from build123d import *

# Parameters (mm, degrees)
BOSS_EXTRUDE1_DEPTH = 2
SKETCH1_3_W         = 70
SKETCH1_3_H         = 43
BOSS_EXTRUDE2_DEPTH = 4
SKETCH1_5_W         = 40
SKETCH1_5_H         = 24
CUT_EXTRUDE4_DEPTH  = 2
CUT_EXTRUDE5_REACH  = 81.505
SKETCH2_W           = 39
SKETCH2_H           = 1.5
BOSS_EXTRUDE3_START = -0.5
BOSS_EXTRUDE3_DEPTH = 0.6
FILLET1_R           = 1


with BuildPart() as part:
    # Sketch1 → Boss-Extrude1 (new body)
    with BuildSketch(Plane(origin=(0, 0, 0), x_dir=(1, 0, 0), z_dir=(0, 1, 0))):
        Polygon((0, 0), (64, 0), (66, 0), (66, -1), (66, -38), (66, -39), (64, -39), (0, -39), align=None)
    extrude(amount=BOSS_EXTRUDE1_DEPTH)

    # Sketch1<3> → Boss-Extrude2 (add)
    with BuildSketch(Plane(origin=(0, 0, 0), x_dir=(1, 0, 0), z_dir=(0, 1, 0))):
        with Locations((33, -19.5)):
            Rectangle(SKETCH1_3_W, SKETCH1_3_H)
        Polygon((0, 0), (64, 0), (66, 0), (66, -1), (66, -38), (66, -39), (64, -39), (0, -39), align=None, mode=Mode.SUBTRACT)
    extrude(amount=BOSS_EXTRUDE2_DEPTH)

    # Sketch1<5> → Cut-Extrude4 (cut)
    with BuildSketch(Plane(origin=(0, 0, 0), x_dir=(1, 0, 0), z_dir=(0, 1, 0))):
        with Locations((20, -27)):
            Rectangle(SKETCH1_5_W, SKETCH1_5_H)
        with BuildLine():
            ThreePointArc((40, -15), (52, -27), (40, -39))
            Line((40, -39), (40, -15))
        make_face()
    extrude(amount=CUT_EXTRUDE4_DEPTH, mode=Mode.SUBTRACT)

    # Sketch2 → Cut-Extrude5 (cut, up to next)
    with BuildSketch(Plane(origin=(0, 0, 0), x_dir=(0, 0, -1), z_dir=(1, 0, 0)), mode=Mode.PRIVATE) as cut_extrude5_sk1:
        with Locations((-19.5, 3.25)):
            Rectangle(SKETCH2_W, SKETCH2_H)
    cut_extrude5_tool1 = extrude(cut_extrude5_sk1.sketch, amount=-CUT_EXTRUDE5_REACH, mode=Mode.PRIVATE) & part.part
    add(cut_extrude5_tool1.solids().sort_by_distance((0, 3.25, 19.5))[0], mode=Mode.SUBTRACT)

    # Sketch3 → Boss-Extrude3 (add)
    with BuildSketch(Plane(origin=(0, 4, 0), x_dir=(1, 0, 0), z_dir=(0, 1, 0)).offset(BOSS_EXTRUDE3_START)):
        Polygon((-2, -41), (68, -41), (68, 2), (-2, 2), (-2, -1), (65, -1), (65, -38), (-2, -38), align=None)
    extrude(amount=BOSS_EXTRUDE3_DEPTH)

    # Fillet1
    fillet1_edges = [part.edges().sort_by_distance(p)[0] for p in [
        (68, 2.05, -2),
        (-2, 0, 19.5),
        (-2, 2.05, -2),
        (33, 0, 41),
        (-2, 2.05, 41),
        (68, 2.05, 41),
        (33, 0, -2),
        (68, 0, 19.5),
        (33, 4.1, 41),
        (68, 4.1, 19.5),
        (33, 4.1, -2),
    ]]
    fillet(fillet1_edges, radius=FILLET1_R)


solid = part.part
Work out the finished part from the listing and answer in its coordinate system (mm). A direction names the side the tool comes from. Round coordinates to 2 decimals unless told otherwise and drop trailing zeros. Write each loop counter-clockwise with the first axis right and the second up, starting at its lowest first coordinate (ties: lowest second). Pieces come first, ordered by that corner, then holes. Notation, with made-up numbers: (77, 25.25) - (96, 25.25) arc R17 cw to (96, 55.25) - close; hole circle Ø7 at (-13.75, 71.5). An arc over 180 degrees is marked (long way). Answer in a Markdown table with one row per item. Add a question column.
1. Given pin 1 (0.5 mm diameter, centred on x = 41, y = 4, fed in from +Z); pin 2 (1.6 mm diameter, centred on x = -1, z = 23.5, fed in from +Y); pin 3 (11.5 mm diameter, centred on x = 16.5, z = 19.5, fed in from +Y), each flat-ended and moving along its own axis, determine where each tip first touches the part or whether it passes through.
2. The mould has two halves that part along X. Classify faces 4 (the flat face through (-2, 2, 20)), 5 (the flat face through (43, 4.1, 39)), 6 (the flat face through (32, 3, 0)): +X half, -X half, draft (parallel to the pull), parting line (faces both ways), or undercut.
3. A cutting plane is placed at A-A, the plane z = 27. Determine the outline of the cut face in (x, y), and give its area (3 significant figures).
4. A cutting plane is placed at C-C, the plane z = 12. Determine the outline of the cut face in (x, y).
5. For faces 1 (the flat face through (31.8, 3.5, 0.6)), 2 (the flat face through (66, 3, 19)), 3 (the flat face through (20, 1, 15)), determine the directions among +Z, -Z, +X, -X, +Y, -Y from which every point of the face is accessible in a straight line to the end or side of a thin tool.
6. Find the intervals of material crossed by line 1 along Z through (x, y) = (2, 0.85); line 2 along Z through (x, y) = (17.5, 3.05); line 3 along Y through (x, z) = (51.5, 8.5), in increasing order. Write a range as from..to.
7. A cutting plane is placed at D-D, the plane x = 44.5. Determine the outline of the cut face in (y, z).
8. A cutting plane is placed at B-B, the plane x = 11. Determine the outline of the cut face in (y, z), and give its area (3 significant figures).
Worked out:
| question | item | result |
|---|---|---|
| 1 | pin 1 | z = 40.76 |
| 1 | pin 2 | y = 2.5 |
| 1 | pin 3 | y = 2 |
| 2 | face 4 | -X half |
| 2 | face 5 | draft |
| 2 | face 6 | undercut |
| 3 | outline | (-2, 1) arc R1 ccw to (-1, 0) - (0, 0) - (0, 2.5) - (-2, 2.5) - close; (52, 0) - (67, 0) arc R1 ccw to (68, 1) - (68, 3.1) arc R1 ccw to (67, 4.1) - (65, 4.1) - (65, 3.5) - (66, 3.5) - (66, 2) - (52, 2) - close |
| 3 | area | 41.2 mm^2 |
| 4 | outline | (-2, 1) arc R1 ccw to (-1, 0) - (67, 0) arc R1 ccw to (68, 1) - (68, 3.1) arc R1 ccw to (67, 4.1) - (65, 4.1) - (65, 3.5) - (66, 3.5) - (66, 2) - (0, 2) - (0, 2.5) - (-2, 2.5) - close |
| 5 | face 1 | -X |
| 5 | face 2 | none |
| 5 | face 3 | +Y, -Y |
| 6 | line 1 | -1.99..15, 39..40.99 |
| 6 | line 2 | -2..0, 39..41 |
| 6 | line 3 | 0..2 |
| 7 | outline | (0, -1) arc R1 ccw to (1, -2) - (3.1, -2) arc R1 ccw to (4.1, -1) - (4.1, 1) - (3.5, 1) - (3.5, 0) - (2, 0) - (2, 15.88) - (0, 15.88) - close; (0, 38.12) - (2, 38.12) - (2, 39) - (3.5, 39) - (3.5, 38) - (4.1, 38) - (4.1, 40) arc R1 ccw to (3.1, 41) - (1, 41) arc R1 ccw to (0, 40) - close |
| 8 | outline | (0, -1) arc R1 ccw to (1, -2) - (3.1, -2) arc R1 ccw to (4.1, -1) - (4.1, 1) - (3.5, 1) - (3.5, 0) - (2, 0) - (2, 15) - (0, 15) - close; (0, 39) - (3.5, 39) - (3.5, 38) - (4.1, 38) - (4.1, 40) arc R1 ccw to (3.1, 41) - (1, 41) arc R1 ccw to (0, 40) - close |
| 8 | area | 46.7 mm^2 |
